```python
from build123d import *

# Parameters (mm, degrees)
SKETCH3_R               = 6.5
CUT_EXTRUDE1_DEPTH      = 19
CUT_EXTRUDE1_DEPTH_BACK = 19
CUT_EXTRUDE2_START      = 10
SKETCH4_R               = 8.5
CUT_EXTRUDE2_DEPTH      = 10
SKETCH5_R               = 5
CUT_EXTRUDE3_DEPTH      = 10
CUT_EXTRUDE4_START      = 12
SKETCH6_R               = 9
CUT_EXTRUDE4_DEPTH      = 12


with BuildPart() as part:
    # Sketch2 → Revolve1 (revolve)
    with BuildSketch(Plane.XY):
        with BuildLine():
            Line((13.416407865, 12), (34.325156356, 10.537917876))
            ThreePointArc((34.325156356, 10.537917876), (46.046347106, 14.963460754), (57.037551508, 8.949712492))
            Line((57.037551508, 8.949712492), (88.873707199, 6.72351162))
            ThreePointArc((88.873707199, 6.72351162), (103.489856271, 12.522815307), (113, 0))
            Line((113, 0), (-18, 0))
            ThreePointArc((-18, 0), (-6.422797616, 16.815102461), (13.416407865, 12))
        make_face()
    revolve(axis=Axis((-18, 0, 0), (1, 0, 0)))

    # Sketch3 → Cut-Extrude1 (cut, two sides)
    with BuildSketch(Plane(origin=(0, 0, 0), x_dir=(1, 0, 0), z_dir=(0, 1, 0))) as cut_extrude1_sk:
        with Locations((45, 0)):
            Circle(SKETCH3_R)
    extrude(amount=CUT_EXTRUDE1_DEPTH, mode=Mode.SUBTRACT)
    extrude(cut_extrude1_sk.sketch, amount=-CUT_EXTRUDE1_DEPTH_BACK, mode=Mode.SUBTRACT)

    # Sketch4 → Cut-Extrude2 (cut)
    with BuildSketch(Plane(origin=(0, 0, 0), x_dir=(1, 0, 0), z_dir=(0, 1, 0)).offset(CUT_EXTRUDE2_START)):
        with Locations((100, 0)):
            Circle(SKETCH4_R)
    extrude(amount=CUT_EXTRUDE2_DEPTH, mode=Mode.SUBTRACT)

    # Sketch5 → Cut-Extrude3 (cut)
    with BuildSketch(Plane(origin=(0, 10, 0), x_dir=(1, 0, 0), z_dir=(0, 1, 0))):
        with Locations((100, 0)):
            Circle(SKETCH5_R)
    extrude(amount=-CUT_EXTRUDE3_DEPTH, mode=Mode.SUBTRACT)

    # Sketch6 → Cut-Extrude4 (cut)
    with BuildSketch(Plane(origin=(0, 0, 0), x_dir=(1, 0, 0), z_dir=(0, 1, 0)).offset(CUT_EXTRUDE4_START)):
        with Locations((45, 0)):
            Circle(SKETCH6_R)
    cut_extrude4 = extrude(amount=CUT_EXTRUDE4_DEPTH, mode=Mode.SUBTRACT)

    # Mirror1: Cut-Extrude4 across plane
    add(cut_extrude4.mirror(Plane.ZX), mode=Mode.SUBTRACT)


solid = part.part
```
Geometry: final body of the model. Coordinates: model frame, mm. A direction names the side the tool comes from. Give positions to 0.01 mm unless a question says otherwise; leave off trailing zeros. Loops run counter-clockwise (first coordinate to the right, second up) from the corner with the lowest first, then second, coordinate; pieces in that order, holes last. Notation, with made-up numbers: (59.25, 54.25) -> (107.25, 54.25) arc R22 cw to (107.25, 68.25) -> close; hole circle Ø5 at (-37, -7). An arc over 180 degrees is marked (long way). Return JSON: item names as keys, results as strings.
Item 1: Access query for faces 1 (the conical face through (73.18, 7.46, 2.35)), 2 (the cylindrical face through (104.619, 5.07, 1.915)), 3 (the cylindrical face through (38.506, 0.168, -0.286)), 4 (the flat face through (48, -12, 6)), 5 (the flat face through (48, 12, 6)). Directions: +Z, -Z, +X, -X, +Y, -Y. A direction counts if a zero-diameter tool reaches every point of the face in a straight line with its end or side. Return the directions, or none.
Filled in:
{"face 1": "none", "face 2": "+Y", "face 3": "+Y, -Y", "face 4": "+Z, -Z, -Y", "face 5": "+Z, -Z, +X, +Y"}
Item 2: Section D-D, the plane y = 3. Count the separate pieces of the cut face and the enclosed holes in it, plus the area to 3 significant figures.
Filled in:
{"separate pieces": "1", "enclosed holes": "2", "area": "2,710 mm^2"}
Item 3: Mould query, pull axis X, two halves, no side actions, for faces 6 (the flat face through (104, 10, 4)), 7 (the flat face through (100, 0, 0)). Classes: released by +X, released by -X, zero draft, split by the parting line, or undercut.
Filled in:
{"face 6": "zero draft", "face 7": "undercut"}
Item 4: Line query: line 1 (X direction, y = 6.5, z = 0); line 2 (X direction, y = 9, z = 3.5); line 3 (X direction, y = 3.5, z = 0). Output: solid intervals per line, ascending.
Filled in:
{"line 1": "-16.79 to 38.5, 51.5 to 95, 105 to 111.26", "line 2": "-15.19 to 39.52, 50.48 to 56.48, 91.3 to 96.43, 103.57 to 108.7", "line 3": "-17.66 to 38.5, 51.5 to 95, 105 to 112.52"}
Item 5: Pin query (flat end, axial travel): P1, Ø8, axis at x = 2.5, z = -2, coming from the -Y side; P2, Ø8, axis at x = 100, z = 0, coming from the +Y side; P3, Ø9, axis at x = 44, z = 1, coming from the +Y side; P4, Ø1, axis at y = 6, z = -12.5, coming from the -X side. Return the tip coordinate at first contact, or that it passes through.
Filled in:
{"P1": "y = -18", "P2": "y = 0", "P3": "through", "P4": "x = -12.06"}
Item 6: Section C-C, the plane x = 100. Output: boundary loops of the cut face in (y, z).
Filled in:
{"outline": "(0, -5) -> (0, 5) -> (10, 5) -> (10, 8.31) arc R13 ccw (long way) to (10, -8.31) -> (10, -5) -> close"}
Item 7: Section A-A, the plane x = 45. Output: boundary loops of the cut face in (y, z).
Filled in:
{"outline": "(-12, -9) arc R15 ccw to (12, -9) -> (12, -6.5) -> (-12, -6.5) -> close; (-12, 6.5) -> (12, 6.5) -> (12, 9) arc R15 ccw to (-12, 9) -> close"}
Item 8: Section B-B, the plane z = 0. Output: boundary loops of the cut face in (x, y).
Filled in:
{"outline": "(13.42, -12) -> (34.33, -10.54) arc R15 ccw to (36, -12) -> (38.5, -12) -> (38.5, 12) -> (36, 12) arc R15 ccw to (34.33, 10.54) -> (13.42, 12) arc R18 ccw (long way) to start; (51.5, -12) -> (54, -12) arc R15 ccw to (57.04, -8.95) -> (88.87, -6.72) arc R13 ccw (long way) to (108.31, 10) -> (105, 10) -> (105, 0) -> (95, 0) -> (95, 10) -> (91.69, 10) arc R13 ccw to (88.87, 6.72) -> (57.04, 8.95) arc R15 ccw to (54, 12) -> (51.5, 12) -> close"}
